The model under review builds one solid part; all positions refer to its coordinate system, in mm. Round coordinates to 2 decimals unless told otherwise and drop trailing zeros. Write each loop counter-clockwise with the first axis right and the second up, starting at its lowest first coordinate (ties: lowest second). Pieces come first, ordered by that corner, then holes. Notation, with made-up numbers: (23, 61.25) - (31, 61.25) arc R24 ccw to (31, 79.25) - close; hole circle Ø4 at (31, -8). An arc over 180 degrees is marked (long way). Return JSON: item names as keys, results as strings.
from build123d import *

# Parameters (mm, degrees)
F0_W        = 168
F0_H        = 95
F0_W_2      = 165
F0_H_2      = 92
F1_DEPTH    = 2.2
F1_FACE_W   = 168
F1_FACE_H   = 95
F1_FACE_W_2 = 165
F1_FACE_H_2 = 92
F2_DEPTH    = 1
F3_R        = 2


with BuildPart() as f1:
    # F0 (on Top) → F1 (new body)
    with BuildSketch(Plane.XY):
        Rectangle(F0_W, F0_H)
        Rectangle(F0_W_2, F0_H_2, mode=Mode.SUBTRACT)
    extrude(amount=F1_DEPTH)

    # F1_face (on face) + F0 (on Top) → F2 (join)
    with BuildSketch(Plane(origin=(0, 0, 0), x_dir=(1, 0, 0), z_dir=(0, 0, -1))):
        Rectangle(F1_FACE_W, F1_FACE_H)
        Rectangle(F1_FACE_W_2, F1_FACE_H_2, mode=Mode.SUBTRACT)
    with BuildSketch(Plane.XY):
        Rectangle(F0_W_2, F0_H_2)
    extrude(amount=F2_DEPTH, dir=(0, 0, -1))

    # F3
    f3_edges = [f1.edges().sort_by_distance(p)[0] for p in [
        (-84, -47.5, 0.6),
        (-84, 47.5, 0.6),
        (84, -47.5, 0.6),
        (84, 47.5, 0.6),
    ]]
    fillet(f3_edges, radius=F3_R)


solid = f1.part
(1) Clearance check with a flat-ended pin moving along its axis: pin 1 Ø3 at (x, y) = (30.5, -28.5) entering from +Z. State where the tip first meets the part, or that it passes through.
Filled in:
{"pin 1": "stops at z = 0"}
(2) Add section A-A (z = 0.75). Write out the cut boundary in (x, y), plus the area to 3 significant figures.
Filled in:
{"outline": "(-84, -45.5) arc R2 ccw to (-82, -47.5) - (82, -47.5) arc R2 ccw to (84, -45.5) - (84, 45.5) arc R2 ccw to (82, 47.5) - (-82, 47.5) arc R2 ccw to (-84, 45.5) - close; hole (-82.5, -46) - (82.5, -46) - (82.5, 46) - (-82.5, 46) - close", "area": "777 mm2"}
(3) Add section C-C (x = -67.5). Write out the cut boundary in (y, z).
Filled in:
{"outline": "(-47.5, -1) - (47.5, -1) - (47.5, 2.2) - (46, 2.2) - (46, 0) - (-46, 0) - (-46, 2.2) - (-47.5, 2.2) - close"}
(4) Mouldability with a two-part tool opening along Y and no side actions: class faces 1 (the flat face through (-1, -47.5, 1)), 2 (the flat face through (-1, 47.5, 1)), 3 (the flat face through (-1, 1, 0)), 4 (the flat face through (-84, 1, 1)) as released by +Y, released by -Y, zero draft, split by the parting line, or undercut.
Filled in:
{"face 1": "released by -Y", "face 2": "released by +Y", "face 3": "undercut", "face 4": "zero draft"}
(5) Add section B-B (y = -1). Write out the cut boundary in (x, z).
Filled in:
{"outline": "(-84, -1) - (84, -1) - (84, 2.2) - (82.5, 2.2) - (82.5, 0) - (-82.5, 0) - (-82.5, 2.2) - (-84, 2.2) - close"}
(6) Wall thickness on line 1 (X direction, y = 31, z = 0.4); line 2 (Y direction, x = 75.5, z = 1.8); line 3 (Z direction, x = 72.5, y = -12): over which ranges is each line inside the solid? List them lowest first.
Filled in:
{"line 1": "x = -84 to -82.5, 82.5 to 84", "line 2": "y = -47.5 to -46, 46 to 47.5", "line 3": "z = -1 to 0"}
